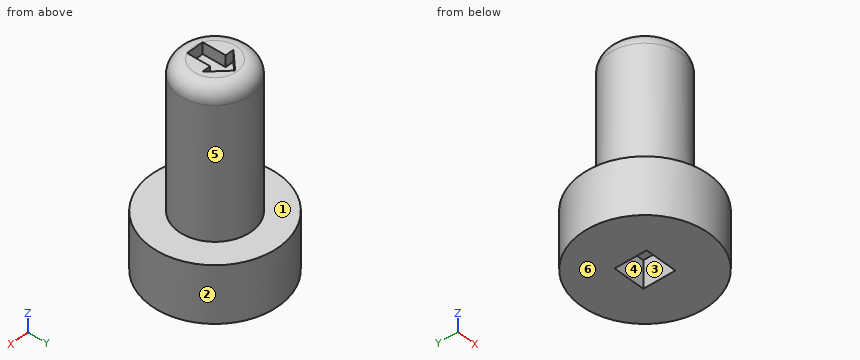
Autodesk Fusion 360 part; units mm, degrees
sketch "Sketch1" plane through (0, 0, 0) normal (0, 0, 1) x (1, 0, 0)
  line L0 (121.4132, 31.9574) -> (124.1913, 31.9574)
  line L1 (124.1913, 31.9574) -> (124.1913, 29.1793)
  line L2 (124.1913, 29.1793) -> (121.4132, 29.1793)
  line L3 (121.4132, 29.1793) -> (121.4132, 31.9574)
  circle A0 centre (122.8023, 30.5684) radius 5.5563
  dimension "d1" = 2.7781
  dimension "d2" = 2.7781
  dimension "d17" = 11.1125
extrude "Extrude1" add sketch "Sketch1" along normal blind 2.3813
extrude "Extrude4" add sketch "Sketch1" along normal blind 2.54 from surface at 2.3813 contours L0 L1 L2 L3 | A0
sketch "Sketch2" plane through (0, 0, 4.9213) normal (0, 0, 1) x (-1, 0, 0)
  line L0 (-124.1913, -29.1793) -> (-121.4132, -29.1793)
  line L1 (-121.4132, -29.1793) -> (-121.4132, -31.9574)
  line L2 (-121.4132, -31.9574) -> (-124.1913, -31.9574)
  line L3 (-124.1913, -31.9574) -> (-124.1913, -29.1793)
  circle A0 centre (-122.8023, -30.5684) radius 3.175
  circle A1 centre (-122.8023, -30.5684) radius 5.5562
  circle A2 centre (-122.8023, -30.5684) radius 5.5562
  point P0 (-121.4132, -30.5684)
  point P1 (-122.8023, -31.9574)
  dimension "d6" = 6.35
extrude "Extrude2" add sketch "Sketch2" along normal blind 12.7 contours L0 L1 L2 L3 | A0
fillet "Fillet1" radius 1.27 1 edges at (125.7624, 31.7165, 17.6213)
sketch "Sketch3" plane through (0, 0, 17.6213) normal (0, 0, 1) x (-1, 0, 0)
  circle A0 centre (-122.8023, -30.5684) radius 1.905
  line L0 (-122.0523, -30.8184) -> (-123.5523, -30.8184) construction
  line L1 (-123.5523, -30.8184) -> (-123.5523, -28.8184)
  line L2 (-123.5523, -28.8184) -> (-122.0523, -28.8184)
  line L3 (-122.0523, -28.8184) -> (-122.0523, -30.8184)
  line L4 (-121.3023, -30.8184) -> (-124.3023, -30.8184)
  line L5 (-124.3023, -30.8184) -> (-122.8023, -32.3184)
  line L6 (-122.8023, -32.3184) -> (-121.3023, -30.8184)
  line L7 (-122.8023, -32.3184) -> (-122.8023, -28.8184) construction
  point P0 (-122.8023, -30.8184)
  point P1 (-122.8023, -30.5684)
  dimension "d11" = 1.5
  dimension "d12" = 2
  dimension "d13" = 1.5
  dimension "d14" = 3
extrude "Extrude3" cut sketch "Sketch3" against normal blind 1 contours L1 L2 L3 L4 | L4 L5 L6
equation "d1 = ( 7 / 64 ) * 1 in"
equation "d2 = ( 7 / 64 ) * 1 in"
equation "d4 = ( 3 / 32 ) * 1 in"
equation "d17 = ( 7 / 16 ) * 1 in"
The model under review builds one solid part; all positions refer to its coordinate system, in mm. Face numbers are marked on the shaded views. A direction names the side the tool comes from. Round coordinates to 2 decimals unless told otherwise and drop trailing zeros. Order: outer loops, then holes, each group sorted by start corner. A loop starts at its lowest first (then second) coordinate and runs counter-clockwise, first axis right, second up. Notation, with made-up numbers: (14, 16) -> (35, 16) arc R6 ccw to (35, 20) -> close; hole circle Ø6 at (-37.75, -15.75). An arc over 180 degrees is marked (long way). Return JSON: item names as keys, results as strings.
1. Take a section at D-D (z = 7.5). Write out the cut boundary in (x, y) (3 decimals).
Answer block:
{"outline": "circle Ø6.35 at (122.802, 30.568)"}
2. Insertion check: P1, Ø3, axis at x = 124.5, z = 12.5, coming from the -Y side; P2, Ø5, axis at y = 30, z = 7.5, coming from the +X side; P3, Ø0.6, axis at x = 124, z = 17.5, coming from the +Y side; P4, Ø1, axis at y = 26.5, z = 12, coming from the +X side (1 decimal). Each pin has a flat end and moves straight along its axis. Give the tip position at first contact, or say it passes through.
Answer block:
{"P1": "stops at y = 27.4", "P2": "stops at x = 125.98", "P3": "stops at y = 33.18", "P4": "passes through"}
3. The part is to be moulded in two halves that separate along X. For the marked faces 3, 4, 5 and 6, say which applies: +X half, -X half, draft (parallel to the pull), parting line (faces both ways), or undercut.
Answer block:
{"face 3": "undercut", "face 4": "undercut", "face 5": "parting line", "face 6": "draft"}
4. For L1, parallel to Z at x = 126.25, y = 30.25; L2, parallel to X at y = 30.5, z = 16.25; L3, parallel to Y at x = 121.5, z = 2.25, list the stretches that pass through material, from the lowest coordinate up. Write a range as [from, to].
Answer block:
{"L1": "z = [0, 4.92]", "L2": "x = [119.63, 125.98]", "L3": "y = [25.17, 29.18], [31.96, 35.97]"}
5. Take a section at A-A (z = 1.25). Write out the cut boundary in (x, y).
Answer block:
{"outline": "circle Ø11.11 at (122.8, 30.57); hole (121.41, 29.18) -> (124.19, 29.18) -> (124.19, 31.96) -> (121.41, 31.96) -> close"}
6. For the marked faces 1 and 2, list the 3-axis set-ups (+Z, -Z, +X, -X, +Y, -Y) from which the entire face can be reached by the end or side of a thin tool; tool diameter is ignored.
Answer block:
{"face 1": "+Z", "face 2": "+Z, -Z"}
7. Take a section at C-C (y = 35.5). Write out the cut boundary in (x, z).
Answer block:
{"outline": "(120.24, 0) -> (125.36, 0) -> (125.36, 4.92) -> (120.24, 4.92) -> close"}
8. Take a section at B-B (x = 118). Write out the cut boundary in (y, z).
Answer block:
{"outline": "(27.77, 0) -> (33.36, 0) -> (33.36, 4.92) -> (27.77, 4.92) -> close"}
